```python
from build123d import *

# Parameters (mm, degrees)
SKETCH1_R               = 6.5
BOSS_EXTRUDE1_DEPTH     = 15
CUT_EXTRUDE1_DEPTH      = 18.592612086
CUT_EXTRUDE1_DEPTH_BACK = 18.592612086
SKETCH2_R               = 1.6383
FILLET1_SIZE            = 1.5


with BuildPart() as part:
    # Sketch1 → Boss-Extrude1 (new body)
    with BuildSketch(Plane(origin=(0, 0, 0), x_dir=(1, 0, 0), z_dir=(0, 1, 0))):
        with Locations(Location((0, 0, 0), (0, 0, 270))):
            Circle(SKETCH1_R)
    extrude(amount=BOSS_EXTRUDE1_DEPTH)

    # Sketch2 → Cut-Extrude1 (cut, two sides: drawn at the far end of the back side and taken through both)
    with BuildSketch(Plane(origin=(0, 15, 0), x_dir=(1, 0, 0), z_dir=(0, 1, 0)).offset(-CUT_EXTRUDE1_DEPTH_BACK)):
        with Locations(Location((0, 0, 0), (0, 0, 270))):
            Circle(SKETCH2_R)
    extrude(amount=CUT_EXTRUDE1_DEPTH + CUT_EXTRUDE1_DEPTH_BACK, mode=Mode.SUBTRACT)

    # Fillet1
    # a fillet whose section is not a circle: 1.5 mm, written as the material it takes off along each edge
    with BuildSketch(Plane(origin=(0, 15, 0), x_dir=(0, 0, 1), z_dir=(-1, 0, 0))) as fillet1_piece_1:
        with BuildLine():
            Bezier((1.6383 + FILLET1_SIZE, 0), (1.6383, 0), (1.6383, -FILLET1_SIZE), weights=[1, 0.106066017, 1])
            Line((1.6383, -FILLET1_SIZE), (1.6383, 0))
            Line((1.6383, 0), (1.6383 + FILLET1_SIZE, 0))
        make_face()
    revolve(axis=Axis((0, 15, 0), (0, 1, 0)), mode=Mode.SUBTRACT)


solid = part.part
```
Design review of the part built by this model. Coordinates are the model's own, in mm. Give positions to 0.01 mm unless a question says otherwise; leave off trailing zeros. Loops run counter-clockwise (first coordinate to the right, second up) from the corner with the lowest first, then second, coordinate; pieces in that order, holes last. Notation, with made-up numbers: (4, -8) -> (29, -8) arc R29 ccw to (29, 20) -> close; hole circle Ø6 at (86, 24.5). An arc over 180 degrees is marked (long way). One line per item, written item: value.
Q1. Draft analysis for pull direction Z (two halves, no side actions). For faces 1 (the cylindrical face through (1.107, 6.656, -1.207)), 2 (the flat face through (2, 15, 3)), 3 (the cylindrical face through (-3.955, 7.395, -5.158)), state which applies: pulls with the +Z half, pulls with the -Z half, needs draft (parallel to the pull), parting line crosses it, or undercut.
Numbers:
face 1: undercut
face 2: needs draft
face 3: parting line crosses it
Q2. For L1, parallel to X at y = 9.75, z = 0; L2, parallel to X at y = 5, z = -1, list the stretches that pass through material, from the lowest coordinate up.
Numbers:
L1: x = -6.5 to -1.64, 1.64 to 6.5
L2: x = -6.42 to -1.3, 1.3 to 6.42
Q3. We need section B-B on x = 5. Give the boundary of the cut face in (y, z).
Numbers:
outline: (0, -4.15) -> (15, -4.15) -> (15, 4.15) -> (0, 4.15) -> close
Q4. We need section C-C on z = -4.5. Give the boundary of the cut face in (x, y), and give its area (3 significant figures).
Numbers:
outline: (-4.69, 0) -> (4.69, 0) -> (4.69, 15) -> (-4.69, 15) -> close
area: 141 mm^2
Q5. For pin 1 Ø4 at (x, y) = (-4.5, 4.5) entering from +Z; pin 2 Ø6 at (y, z) = (7, -5) entering from +X; pin 3 Ø2 at (y, z) = (8, -4) entering from +X, all flat-tipped, find the tip position at first contact; note any pin that passes through.
Numbers:
pin 1: stops at z = 6
pin 2: stops at x = 6.18
pin 3: stops at x = 5.77
Q6. We need section A-A on y = 9.5. Give the boundary of the cut face in (x, z), and give its area (3 significant figures).
Numbers:
outline: circle Ø13 at (0, 0); hole circle Ø3.28 at (0, 0)
area: 124 mm^2
